Geometry check sheet. Reference: the model listing, model coordinates, mm. A direction names the side the tool comes from. Give positions to 0.01 mm unless a question says otherwise; leave off trailing zeros. Loops run counter-clockwise (first coordinate to the right, second up) from the corner with the lowest first, then second, coordinate; pieces in that order, holes last. Notation, with made-up numbers: (56, 48) -> (81, 48) arc R22 cw to (81, 68) -> close; hole circle Ø4 at (27, 19.5). An arc over 180 degrees is marked (long way). One line per item, written item: value. Start each with the question number.
(1) Scan lines: line 1 along X through (y, z) = (1.45, 15); line 2 along Y through (x, z) = (24, 12); line 3 along Y through (x, z) = (5, 15). Record each from-to range of solid material in increasing order. Write a range as from..to.
(2) Tool access check on faces 5 (the face through (20, 4, 24)), 6 (the face through (14.76, 14.75, 14.96)), 7 (the face through (14.9, 3.2, 15)). Record the directions out of +Z, -Z, +X, -X, +Y, -Y that give a thin tool (end or side, any length) a straight path to the whole face; none if there is none.
(3) Draft check along Z on faces 1 (the face through (15, 16, 29)), 2 (the face through (15, 17, 2)), 3 (the face through (20, 14, 24)), 4 (the face through (27.7, 14.75, 14.96)). Enter one of: pulls with the +Z half, pulls with the -Z half, needs draft (parallel to the pull), parting line crosses it, or undercut.
(4) Sectioned sample at C-C, the plane x = 23. Record the cut outline in (y, z), then the cut area to 3 significant figures.
(5) Sectioned sample at A-A, the plane y = 9. Record the cut outline in (x, z).
(6) Sectioned sample at B-B, the plane z = 15. Record the cut outline in (x, y), then the cut area to 4 significant figures.
(7) Gauge pin test, flat ends, axial feed: pin 1 Ø5.5 at (x, z) = (23, 15) entering from -Y; pin 2 Ø5 at (x, y) = (25, 4) entering from +Z. Record the tip position at first contact, or that the pin passes through.
(8) Sectioned sample at D-D, the plane x = 11.5. Record the cut outline in (y, z), then the cut area to 3 significant figures.
from build123d import *

# Parameters (mm, degrees)
ESQUISSE1_W                        = 30
ESQUISSE1_H                        = 30
BOSS_EXTRU_1_DEPTH                 = 4
ENL_V_MAT_EXTRU_1_DEPTH            = 12.400000001
ESQUISSE3_W                        = 10
ESQUISSE3_H                        = 30
BOSS_EXTRU_2_DEPTH                 = 14
ESQUISSE4_W                        = 30
ESQUISSE4_H                        = 4
BOSS_EXTRU_3_DEPTH                 = 20
ESQUISSE5_R                        = 5.75
ENL_V_MAT_EXTRU_2_DEPTH            = 20
DIAM_TRE_DU_PER_AGE_6_0_6_1_REACH  = 20
DIAM_TRE_DU_PER_AGE_6_0_6_1_BORE_R = 3
DIAM_TRE_DU_PER_AGE_6_0_6_2_D      = 6
DIAM_TRE_DU_PER_AGE_6_0_6_2_DEPTH  = 18
CONG_2_R                           = 5


with BuildPart() as part:
    # Esquisse1 → Boss.-Extru.1 (new body)
    with BuildSketch(Plane.XZ):
        with Locations((15, 15)):
            Rectangle(ESQUISSE1_W, ESQUISSE1_H)
    extrude(amount=-BOSS_EXTRU_1_DEPTH)

    # Esquisse2 → Enlèv. mat.-Extru.1 (cut)
    with BuildSketch(Plane(origin=(22.400000001, 0, 0), x_dir=(0, 0, -1), z_dir=(1, 0, 0))):
        with BuildLine():
            Line((-12.060612309, 4), (-17.939387691, 4))
            ThreePointArc((-17.939387691, 4), (-15, 3.2), (-12.060612309, 4))
        make_face()
    extrude(amount=-ENL_V_MAT_EXTRU_1_DEPTH, mode=Mode.SUBTRACT)

    # Esquisse3 → Boss.-Extru.2 (add)
    with BuildSketch(Plane(origin=(0, 4, 0), x_dir=(-1, 0, 0), z_dir=(0, 1, 0))):
        with Locations((-5, 15)):
            Rectangle(ESQUISSE3_W, ESQUISSE3_H)
    extrude(amount=BOSS_EXTRU_2_DEPTH)

    # Esquisse4 → Boss.-Extru.3 (add)
    with BuildSketch(Plane(origin=(10, 0, 0), x_dir=(0, 0, -1), z_dir=(1, 0, 0))):
        with Locations((-15, 16)):
            Rectangle(ESQUISSE4_W, ESQUISSE4_H)
    extrude(amount=BOSS_EXTRU_3_DEPTH)

    # Esquisse5 → Enlèv. mat.-Extru.2 (cut)
    with BuildSketch(Plane(origin=(30, 0, 0), x_dir=(0, 0, -1), z_dir=(1, 0, 0))):
        with Locations((-15, 9)):
            Circle(ESQUISSE5_R)
    extrude(amount=-ENL_V_MAT_EXTRU_2_DEPTH, mode=Mode.SUBTRACT)

    # Esquisse7 → Enlèvement de matière-Révolution1 (revolve, cut)
    with BuildSketch(Plane(origin=(0, 0, 15), x_dir=(-1, 0, 0), z_dir=(0, 0, -1)), mode=Mode.PRIVATE) as enl_vement_de_mati_re_r_volution1_sk:
        Polygon((-10, 14.75), (-10, 9), (0, 9), (0, 11.75), (-7, 11.75), align=None)
    revolve(enl_vement_de_mati_re_r_volution1_sk.sketch.rotate(Axis((10, 9, 15), (-1, 0, 0)), 29.591845794), axis=Axis((10, 9, 15), (-1, 0, 0)), mode=Mode.SUBTRACT)  # turned: the seam where the file's is

    # Diamètre du perçage Ø6.0 (6)1 bore → Diamètre du perçage Ø6.0 (6)1 (cut, up to next)
    with BuildSketch(Plane(origin=(0, 18, 0), x_dir=(1, 0, 0), z_dir=(0, 1, 0)), mode=Mode.PRIVATE) as diam_tre_du_per_age_6_0_6_1_sk1:
        with Locations((23, -15)):
            Circle(DIAM_TRE_DU_PER_AGE_6_0_6_1_BORE_R)
    diam_tre_du_per_age_6_0_6_1_tool1 = extrude(diam_tre_du_per_age_6_0_6_1_sk1.sketch, amount=-DIAM_TRE_DU_PER_AGE_6_0_6_1_REACH, mode=Mode.PRIVATE) & part.part
    add(diam_tre_du_per_age_6_0_6_1_tool1.solids().sort_by_distance((23, 18, 15))[0], mode=Mode.SUBTRACT)

    # Diamètre du perçage Ø6.0 (6)2
    with Locations(Plane(origin=(0, 0, 0), x_dir=(-1, 0, 0), z_dir=(0, -1, 0))):
        with Locations((-23, -15)):
            Hole(DIAM_TRE_DU_PER_AGE_6_0_6_2_D / 2, depth=DIAM_TRE_DU_PER_AGE_6_0_6_2_DEPTH)

    # Congé2
    cong_2_edges = [part.edges().sort_by_distance(p)[0] for p in [
        (15, 18, 0),
        (15, 0, 0),
        (15, 0, 30),
        (15, 18, 30),
    ]]
    fillet(cong_2_edges, radius=CONG_2_R)


solid = part.part
Calculated:
1. line 1: x = 0..20, 26..30
1. line 2: y = 0..4, 14..18
1. line 3: y = 0..6.25, 11.75..18
2. face 5: +Z, -Z, +X
2. face 6: +X
2. face 7: none
3. face 1: pulls with the +Z half
3. face 2: pulls with the -Z half
3. face 3: needs draft
3. face 4: undercut
4. outline: (0, 5) arc R5 ccw to (4, 0.1) -> (4, 12) -> (0, 12) -> close; (0, 18) -> (4, 18) -> (4, 29.9) arc R5 ccw to (0, 25) -> close; (14, 0.1) arc R5 ccw to (18, 5) -> (18, 12) -> (14, 12) -> close; (14, 18) -> (18, 18) -> (18, 25) arc R5 ccw to (14, 29.9) -> close
4. area: 171 mm2
5. outline: (0, 0) -> (10, 0) -> (10, 9.25) -> (7, 12.25) -> (0, 12.25) -> close; (0, 17.75) -> (7, 17.75) -> (10, 20.75) -> (10, 30) -> (0, 30) -> close
6. outline: (0, 0) -> (20, 0) -> (20, 3.2) -> (10, 3.2) -> (10, 3.25) -> (7, 6.25) -> (0, 6.25) -> close; (0, 11.75) -> (7, 11.75) -> (10, 14.75) -> (20, 14.75) -> (20, 18) -> (0, 18) -> close; (26, 0) -> (30, 0) -> (30, 3.25) -> (26, 3.25) -> close; (26, 14.75) -> (30, 14.75) -> (30, 18) -> (26, 18) -> close
6. area: 206.5 mm2
7. pin 1: passes through
7. pin 2: stops at z = 29.9
8. outline: (0, 5) arc R5 ccw to (4, 0.1) -> (4, 12.06) arc R5.8 cw to (4, 17.94) -> (4, 29.9) arc R5 ccw to (0, 25) -> close; (14, 0.1) arc R5 ccw to (18, 5) -> (18, 25) arc R5 ccw to (14, 29.9) -> (14, 17.84) arc R5.75 cw to (14, 12.16) -> close
8. area: 213 mm2
